Check sheet for the drawn part. Datum: minimum x, y, z corner. Units: mm. A direction names the side the tool comes from. Coordinates: 2 decimals unless noted, no trailing zeros. Write each loop counter-clockwise with the first axis right and the second up, starting at its lowest first coordinate (ties: lowest second). Pieces come first, ordered by that corner, then holes. Notation, with made-up numbers: M 67,80.25 L 115,80.25 A23 cw 115,118.25 Z; hole C -16,-31 d2. An arc over 180 degrees is marked long. Answer in a Markdown table with one row per item.
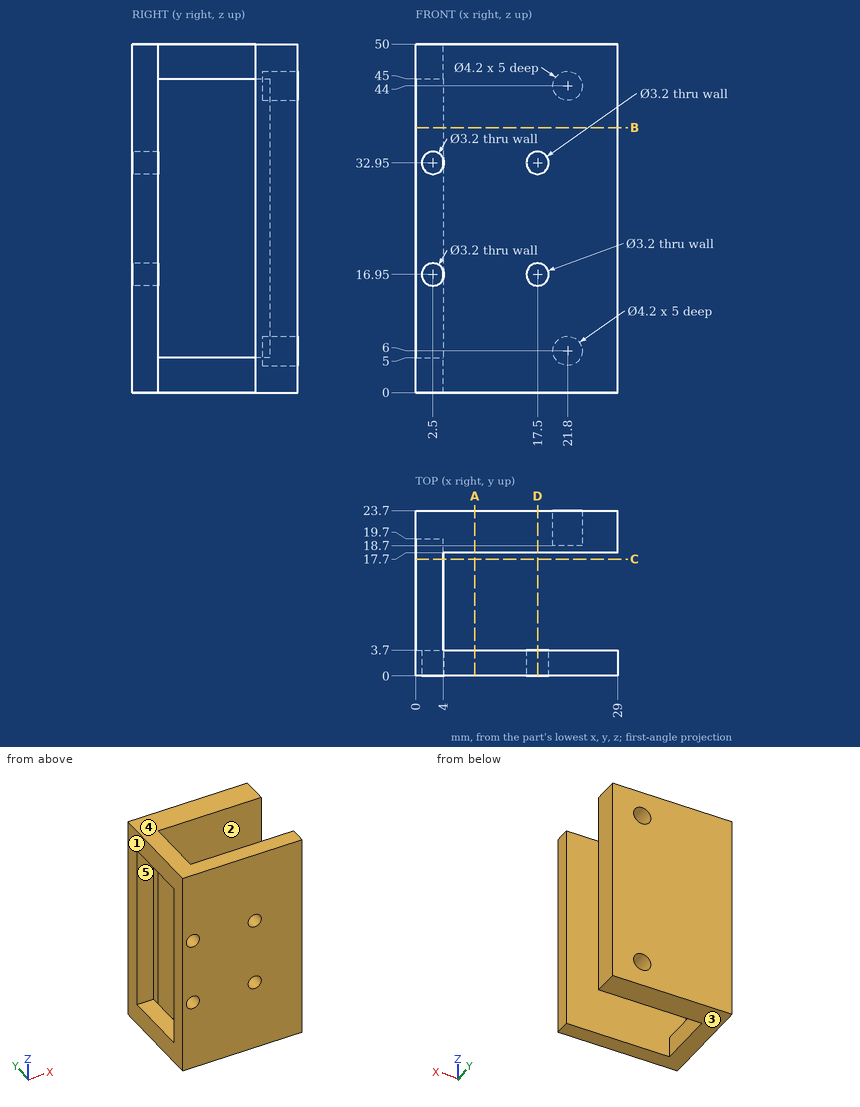
1) Thickness scan on L1, parallel to Z at x = 21.8, y = 22.4; L2, parallel to Z at x = 17.5, y = 1; L3, parallel to Y at x = 26.5, z = 18. Record the ranges inside material, lowest first. Write a range as [from, to].
Response values:
| item | result |
|---|---|
| L1 | z = [0, 3.9], [8.1, 41.9], [46.1, 50] |
| L2 | z = [0, 15.35], [18.55, 31.35], [34.55, 50] |
| L3 | y = [0, 3.7], [17.7, 23.7] |
2) Release check for a two-part mould opening along Z. For the marked faces 3, 4 and 5 record: +Z half, -Z half, draft (parallel to the pull), parting line (faces both ways), or undercut.
Response values:
| item | result |
|---|---|
| face 3 | -Z half |
| face 4 | +Z half |
| face 5 | undercut |
3) Sectioned sample at B-B (z = 38). Record the cut outline in (x, y).
Response values:
| item | result |
|---|---|
| outline | M 0,0 L 29,0 L 29,3.7 L 0,3.7 Z; M 0,19.7 L 4,19.7 L 4,17.7 L 29,17.7 L 29,23.7 L 0,23.7 Z |
4) Tool access check on the marked faces 1 and 2. Record the directions out of +Z, -Z, +X, -X, +Y, -Y that give a thin tool (end or side, any length) a straight path to the whole face; none if there is none.
Response values:
| item | result |
|---|---|
| face 1 | +Z, -Z, -X, +Y, -Y |
| face 2 | +Z, -Z, +X |
5) Sectioned sample at D-D (x = 17.5). Record the cut outline in (y, z), then the cut area to 3 significant figures.
Response values:
| item | result |
|---|---|
| outline | M 0,0 L 3.7,0 L 3.7,15.35 L 0,15.35 Z; M 0,18.55 L 3.7,18.55 L 3.7,31.35 L 0,31.35 Z; M 0,34.55 L 3.7,34.55 L 3.7,50 L 0,50 Z; M 17.7,0 L 23.7,0 L 23.7,50 L 17.7,50 Z |
| area | 461 mm² |
6) Sectioned sample at C-C (y = 16.75). Record the cut outline in (x, z), then the cut area to 3 significant figures.
Response values:
| item | result |
|---|---|
| outline | M 0,0 L 4,0 L 4,5 L 0,5 Z; M 0,45 L 4,45 L 4,50 L 0,50 Z |
| area | 40.0 mm² |
7) Depth check by flat-ended pin: pin 1 (1.6 mm diameter, centred on y = 18.5, z = 26, fed in from -X); pin 2 (4 mm diameter, centred on y = 9, z = 2, fed in from +X); pin 3 (1.3 mm diameter, centred on x = 22.5, z = 43.5, fed in from +Y). Enter the tip coordinate at first touch or a pass-through.
Response values:
| item | result |
|---|---|
| pin 1 | stops at x = 4 |
| pin 2 | stops at x = 4 |
| pin 3 | stops at y = 18.7 |
8) Sectioned sample at A-A (x = 8.5). Record the cut outline in (y, z), then the cut area to 3 significant figures.
Response values:
| item | result |
|---|---|
| outline | M 0,0 L 3.7,0 L 3.7,50 L 0,50 Z; M 17.7,0 L 23.7,0 L 23.7,50 L 17.7,50 Z |
| area | 485 mm² |
